Source: CAD feature listing. Evaluate the final solid. Frame: model axes, mm. Coordinates: 2 decimals unless noted, no trailing zeros. Write each loop counter-clockwise with the first axis right and the second up, starting at its lowest first coordinate (ties: lowest second). Pieces come first, ordered by that corner, then holes. Notation, with made-up numbers: (26.25, 80) - (84.25, 80) arc R8 ccw to (84.25, 84) - close; hole circle Ø6 at (-31.75, 82). An arc over 180 degrees is marked (long way). One line per question, with ' | ' between items.
from build123d import *

# Parameters (mm, degrees)
ESBO_O1_W                  = 74
ESBO_O1_H                  = 77
RESSALTO_EXTRUS_O1_DEPTH   = 2
CORTE_EXTRUS_O1_DEPTH      = 1
CORTE_EXTRUS_O1_DEPTH_BACK = 3
FILETE1_R                  = 10
FILETE2_R                  = 10
FILETE3_R                  = 10


with BuildPart() as part:
    # Esboço1 → Ressalto-extrusão1 (new body)
    with BuildSketch(Plane.XY):
        with Locations((-49.165685596, 5.526315789)):
            Rectangle(ESBO_O1_W, ESBO_O1_H)
    extrude(amount=RESSALTO_EXTRUS_O1_DEPTH)

    # Esboço2 → Corte-extrusão1 (cut, two sides)
    with BuildSketch(Plane.XY.offset(2)) as corte_extrus_o1_sk:
        Polygon((69.094880688, -170.414331392), (-51.165685596, -32.973684211), (-86.165685596, 7.026315789), (-206.426251879, 144.46696297), (-481.307546241, -96.054169596), (-205.786413674, -410.935463958), align=None)
    extrude(amount=CORTE_EXTRUS_O1_DEPTH, mode=Mode.SUBTRACT)
    extrude(corte_extrus_o1_sk.sketch, amount=-CORTE_EXTRUS_O1_DEPTH_BACK, mode=Mode.SUBTRACT)

    # Filete1
    filete1_edges = [part.edges().sort_by_distance(p)[0] for p in [
        (-86.165685596, 7.026315789, 1),
    ]]
    fillet(filete1_edges, radius=FILETE1_R)

    # Filete2
    filete2_edges = [part.edges().sort_by_distance(p)[0] for p in [
        (-51.165685596, -32.973684211, 1),
    ]]
    fillet(filete2_edges, radius=FILETE2_R)

    # Filete3
    filete3_edges = [part.edges().sort_by_distance(p)[0] for p in [
        (-12.165685596, 44.026315789, 1),
    ]]
    fillet(filete3_edges, radius=FILETE3_R)


solid = part.part
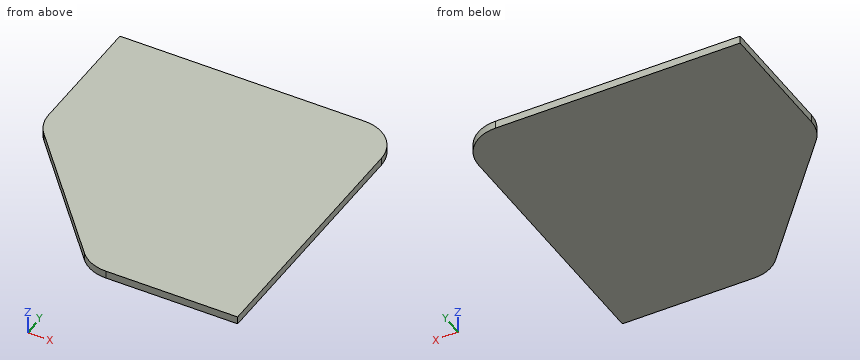
Item 1: Ray query, line 1 along Y through (x, z) = (-67, 1.65); line 2 along X through (y, z) = (7.5, 1.9); line 3 along X through (y, z) = (-21, 0.2). Return the intervals inside material, ascending. Write a range as [from, to].
Check sheet entries:
line 1: [-14.88, 44.03] | line 2: [-85.61, -12.17] | line 3: [-61.64, -12.17]
Item 2: Pin query (flat end, axial travel): pin 1 Ø1 at (x, z) = (-58.5, 0.5) entering from -Y. Return the tip coordinate at first contact, or that it passes through.
Check sheet entries:
pin 1: y = -25.16
Item 3: Cut plane B-B on y = -7. Return loops of the section in (x, z).
Check sheet entries:
outline: (-73.89, 0) - (-12.17, 0) - (-12.17, 2) - (-73.89, 2) - close
Item 4: Cut plane C-C on x = -72. Return loops of the section in (y, z).
Check sheet entries:
outline: (-9.16, 0) - (44.03, 0) - (44.03, 2) - (-9.16, 2) - close
Item 5: Cut plane A-A on z = 0.45. Return loops of the section in (x, y), and give its area (3 significant figures).
Check sheet entries:
outline: (-86.17, 10.78) arc R10 ccw to (-83.69, 4.2) - (-54.15, -29.56) arc R10 ccw to (-46.63, -32.97) - (-12.17, -32.97) - (-12.17, 34.03) arc R10 ccw to (-22.17, 44.03) - (-86.17, 44.03) - close | area: 4,970 mm²
